from build123d import *

# Parameters (mm, degrees)
F0_W     = 60
F0_H     = 90
F1_DEPTH = 50
F2_R     = 10
F3_DEPTH = 30
F5_DEPTH = 30


with BuildPart() as f1:
    # F0 (on Top) → F1 (new body)
    with BuildSketch(Plane.XY):
        Rectangle(F0_W, F0_H)
    extrude(amount=F1_DEPTH)

    # F2 (on face) → F3 (join)
    with BuildSketch(Plane.XY.offset(50)):
        with Locations((11, 32)):
            Circle(F2_R)
        with Locations((-16, 27)):
            Circle(F2_R)
        with BuildLine():
            add(Edge.make_bspline(
                [(2.990381, -27.5), (6.02147, -22.25), (-14.979646, -13.625), (-35.980762, -5), (-18.010735, -18.875), (-0.040708, -32.75), (2.990381, -27.5)],
                knots=[0, 0, 0, 2.094395, 2.094395, 4.18879, 4.18879, 6.283185, 6.283185, 6.283185], degree=2, weights=[1, 0.5, 1, 0.5, 1, 0.5, 1]))
        make_face()
    extrude(amount=F3_DEPTH)

    # F4 (on face) → F5 (cut)
    with BuildSketch(Plane(origin=(0, 45, 0), x_dir=(-1, 0, 0), z_dir=(0, 1, 0))):
        Polygon((5, 17.928932), (12.071068, 25), (12.071068, 35), (5, 42.071068), (-5, 42.071068), (-12.071068, 35), (-12.071068, 25), (-5, 17.928932), align=None)
    extrude(amount=-F5_DEPTH, mode=Mode.SUBTRACT)


solid = f1.part
CAD build for the part. Positions are in the model's coordinates, mm. A direction names the side the tool comes from. Coordinates: 2 decimals unless noted, no trailing zeros. Write each loop counter-clockwise with the first axis right and the second up, starting at its lowest first coordinate (ties: lowest second). Pieces come first, ordered by that corner, then holes. Notation, with made-up numbers: (74, 69) - (130, 69) arc R21 ccw to (130, 107) - close; hole circle Ø7 at (64.25, 0.5). An arc over 180 degrees is marked (long way). Use a Markdown table: item, result. Add a question column.
Item 1: Band-saw the part on A-A, the plane z = 32.5. Give the cut face in (x, y), and give its area (3 significant figures).
Item 2: Mould opens along X. For faces 1 (the face through (11, 32, 80)), 2 (the face through (-8.585, 30.21, 38.486)), 3 (the face through (-30, -1, 25)) say: pulls with the +X half, pulls with the -X half, needs draft (parallel to the pull), parting line crosses it, or undercut.
Item 3: Flat gauge pins, fed straight in: pin 1 (3 mm diameter, centred on x = 15, y = 20.5, fed in from +Z); pin 2 (12 mm diameter, centred on x = 18.5, z = 67.5, fed in from -Y). Where does each tip first touch, or does it go through?
Item 4: Band-saw the part on B-B, the plane x = 15. Give the cut face in (y, z).
Item 5: Drill centre lines: L1, parallel to Z at x = 2.5, y = 33; L2, parallel to Z at x = -3, y = 35; L3, parallel to X at y = 17.5, z = 33. Where is each one in solid material? Low to high. Write a range as from..to.
Item 6: 3-axis set-ups, long thin cutter, end or side, ignore diameter. For faces 4 (the face through (-6.763, 23.17, 64.79)), 5 (the face through (-7, 45, 19)), 6 (the face through (0, 15, 30)): which of +Z, -Z, +X, -X, +Y, -Y reach the whole face in a straight line?
Item 7: Band-saw the part on C-C, the plane y = 27. Give the cut face in (x, z).
Item 8: Band-saw the part on D-D, the plane z = 67.5. Give the number of separate pieces and of enclosed holes in the cut face, and give its area (3 significant figures).
Numbers:
| question | item | result |
|---|---|---|
| 1 | outline | (-30, -45) - (30, -45) - (30, 45) - (12.07, 45) - (12.07, 15) - (-12.07, 15) - (-12.07, 45) - (-30, 45) - close |
| 1 | area | 4,680 mm2 |
| 2 | face 1 | needs draft |
| 2 | face 2 | undercut |
| 2 | face 3 | pulls with the -X half |
| 3 | pin 1 | z = 50 |
| 3 | pin 2 | y = 22.11 |
| 4 | outline | (-45, 0) - (45, 0) - (45, 50) - (41.17, 50) - (41.17, 80) - (22.83, 80) - (22.83, 50) - (-45, 50) - close |
| 5 | L1 | 0..17.93, 42.07..80 |
| 5 | L2 | 0..17.93, 42.07..50 |
| 5 | L3 | -30..-12.07, 12.07..30 |
| 6 | face 4 | +Z |
| 6 | face 5 | +Z, -Z, +X, -X, +Y |
| 6 | face 6 | +Y |
| 7 | outline | (-30, 0) - (30, 0) - (30, 50) - (19.66, 50) - (19.66, 80) - (2.34, 80) - (2.34, 50) - (-6, 50) - (-6, 80) - (-26, 80) - (-26, 50) - (-30, 50) - close; hole (-12.07, 25) - (-5, 17.93) - (5, 17.93) - (12.07, 25) - (12.07, 35) - (5, 42.07) - (-5, 42.07) - (-12.07, 35) - close |
| 8 | separate pieces | 3 |
| 8 | enclosed holes | 0 |
| 8 | area | 793 mm2 |
